from build123d import *

# Parameters (mm, degrees)
EXTRUDE_1_DEPTH     = 40
CUT_EXTRUDE_1_DEPTH = 28


with BuildPart() as part:
    # 草图1 → 凸台-拉伸1 (new, symmetric)
    with BuildSketch(Plane(origin=(0, 0, 0), x_dir=(0, 0, -1), z_dir=(1, 0, 0))):
        Polygon((55, 0), (-55, 0), (-55, 15), (-7.5, 15), (-7.5, 279.793839815), (-32.5, 250), (-39.027036447, 250), (89.530485491, 403.208888624), (96.057521937, 403.208888624), (7.5, 297.670143704), (7.5, 15), (55, 15), align=None)
    extrude(amount=EXTRUDE_1_DEPTH, both=True)

    # 草图2 → 切除-拉伸1 (cut)
    with BuildSketch(Plane(origin=(40, 0, 0), x_dir=(0, 0, -1), z_dir=(1, 0, 0))):
        Polygon((-7.5, 279.793839815), (7.5, 297.670143704), (7.5, 15), (-7.5, 15), align=None)
    cut_extrude_1 = extrude(amount=-CUT_EXTRUDE_1_DEPTH, mode=Mode.SUBTRACT)

    # 镜向1: 切除-拉伸1 across plane
    add(cut_extrude_1.mirror(Plane(origin=(0, 0, 0), x_dir=(0, 0, 1), z_dir=(1, 0, 0))), mode=Mode.SUBTRACT)


solid = part.part
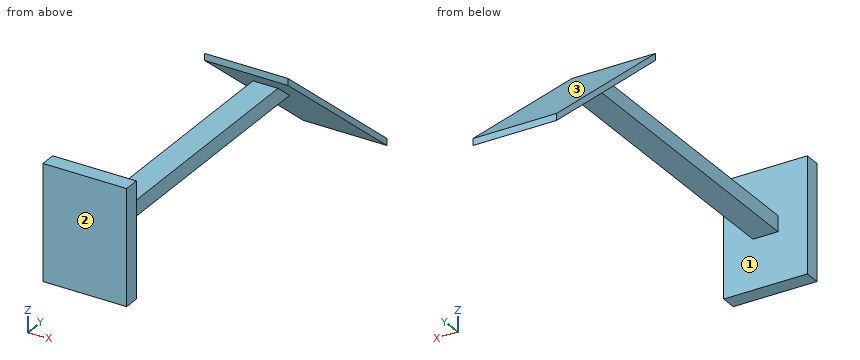
Geometry check sheet. Reference: the model listing, model coordinates, mm. Face numbers are marked on the shaded views. Give positions to 0.01 mm unless a question says otherwise; leave off trailing zeros. Write each loop counter-clockwise with the first axis right and the second up, starting at its lowest first coordinate (ties: lowest second). Pieces come first, ordered by that corner, then holes.
1) Thickness scan on line 1 (Y direction, x = -18.5, z = -15.5); line 2 (Y direction, x = -16.5, z = 1.5); line 3 (Y direction, x = -16.5, z = 40.5). Record the ranges inside material, lowest first.
Values follow:
line 1: y = 0 to 15, 307.2 to 314.98
line 2: y = 0 to 15, 286.94 to 294.72
line 3: y = 0 to 15
2) Go/stop test with flat-tipped pins: pin 1 Ø3.5 at (x, z) = (5.5, 34) entering from -Y; pin 2 Ø4 at (x, y) = (12.5, 163) entering from +Z; pin 3 Ø4 at (x, y) = (12, 342) entering from +Z; pin 4 Ø8 at (x, y) = (-11.5, 207.5) entering from -Z. Record where each tip stops, or that it passes through.
Values follow:
pin 1: stops at y = 0
pin 2: stops at z = 7.5
pin 3: stops at z = -36.49
pin 4: stops at z = -7.5
3) Cross-section at C-C (x = -7). Record the boundary of the cut face in (y, z).
Values follow:
outline: (0, -55) - (15, -55) - (15, -7.5) - (297.67, -7.5) - (403.21, -96.06) - (403.21, -89.53) - (250, 39.03) - (250, 32.5) - (279.79, 7.5) - (15, 7.5) - (15, 55) - (0, 55) - close
4) Cross-section at A-A (x = 22.5). Record the boundary of the cut face in (y, z).
Values follow:
outline: (0, -55) - (15, -55) - (15, 55) - (0, 55) - close; (250, 32.5) - (403.21, -96.06) - (403.21, -89.53) - (250, 39.03) - close
5) Release check for a two-part mould opening along Y. For the marked faces 1, 2 and 3 record: released by +Y, released by -Y, zero draft, split by the parting line, or undercut.
Values follow:
face 1: undercut
face 2: released by -Y
face 3: released by +Y
6) Cross-section at B-B (z = -48.5). Record the boundary of the cut face in (x, y), plus the area to 3 significant figures.
Values follow:
outline: (-40, 0) - (40, 0) - (40, 15) - (-40, 15) - close; (-40, 346.53) - (40, 346.53) - (40, 354.31) - (-40, 354.31) - close
area: 1,820 mm2
7) Cross-section at D-D (y = 239). Record the boundary of the cut face in (x, z).
Values follow:
outline: (-12, -7.5) - (12, -7.5) - (12, 7.5) - (-12, 7.5) - close
